Here's how the part is built. I have some questions about the finished solid (model axes, mm). A direction names the side the tool comes from. Round coordinates to 2 decimals unless told otherwise and drop trailing zeros. Order: outer loops, then holes, each group sorted by start corner. A loop starts at its lowest first (then second) coordinate and runs counter-clockwise, first axis right, second up. Notation, with made-up numbers: (71.25, 10.5) -> (125.25, 10.5) arc R36 ccw to (125.25, 48.5) -> close; hole circle Ø7 at (-1.75, 87). An arc over 180 degrees is marked (long way). One line per item, written item: value.
```python
from build123d import *

# Parameters (mm, degrees)
SKETCH_1_R          = 8
EXTRUDE_1_DEPTH     = 10
SKETCH_2_R          = 5
EXTRUDE_2_DEPTH     = 42
SKETCH_3_R          = 3.5
EXTRUDE_3_DEPTH     = 12
CUT_EXTRUDE_1_DEPTH = 10


with BuildPart() as part:
    # Эскиз1 → Бобышка-Вытянуть1 (new body)
    with BuildSketch(Plane(origin=(0, 0, 0), x_dir=(1, 0, 0), z_dir=(0, 1, 0))):
        Circle(SKETCH_1_R)
    extrude(amount=EXTRUDE_1_DEPTH)

    # Эскиз2 → Бобышка-Вытянуть2 (add)
    with BuildSketch(Plane(origin=(0, 10, 0), x_dir=(1, 0, 0), z_dir=(0, 1, 0))):
        Circle(SKETCH_2_R)
    extrude(amount=EXTRUDE_2_DEPTH)

    # Эскиз3 → Бобышка-Вытянуть3 (add)
    with BuildSketch(Plane(origin=(0, 52, 0), x_dir=(1, 0, 0), z_dir=(0, 1, 0))):
        Circle(SKETCH_3_R)
    extrude(amount=EXTRUDE_3_DEPTH)

    # Эскиз4 → Вырез-Вытянуть1 (cut)
    with BuildSketch(Plane(origin=(0, 0, 0), x_dir=(0, 0, -1), z_dir=(1, 0, 0))):
        with BuildLine():
            Line((-2, 42), (-2, 48))
            ThreePointArc((-2, 48), (0, 50), (2, 48))
            Line((2, 48), (2, 42))
            ThreePointArc((2, 42), (0, 40), (-2, 42))
        make_face()
    extrude(amount=-CUT_EXTRUDE_1_DEPTH, mode=Mode.SUBTRACT)


solid = part.part
```
Q1. I want a section at C-C on y = 7. Write out the boundary of the cut face in (x, z), then the cut area to 3 significant figures.
Answers:
outline: circle Ø16 at (0, 0)
area: 201 mm2
Q2. If we mould it in two halves opening along Z, with no side actions, what happens to faces 4 (the face through (0, 45, 0)), 5 (the face through (-2, 40, 0)), 6 (the face through (0, 64, 0)), 7 (the face through (4.77, 30.71, -1.5))? For each: pulls with the +Z half, pulls with the -Z half, needs draft (parallel to the pull), parting line crosses it, or undercut.
Answers:
face 4: undercut
face 5: undercut
face 6: needs draft
face 7: parting line crosses it
Q3. I need wall thicknesses on line 1 along Y through (x, z) = (-2.5, 3.5); line 2 along Y through (x, z) = (7.5, 0); line 3 along X through (y, z) = (7, -3.5). Which ranges of each line are inside material? Lowest first, please.
Answers:
line 1: 0 to 52
line 2: 0 to 10
line 3: -7.19 to 7.19
Q4. Which directions (+Z, -Z, +X, -X, +Y, -Y) give clear straight access to the entire face, cutting with the end or side of a thin tool? Please do faces 1 (the face through (-2, 45, -2)), 2 (the face through (0, 0, 0)), 3 (the face through (5.2, 10, -0.1)).
Answers:
face 1: -X
face 2: +Z, -Z, +X, -X, -Y
face 3: +Y
Q5. I want a section at D-D on z = 6. Write out the boundary of the cut face in (x, y), then the cut area to 3 significant figures.
Answers:
outline: (-5.29, 0) -> (5.29, 0) -> (5.29, 10) -> (-5.29, 10) -> close
area: 106 mm2
Q6. I want a section at B-B on x = -2.5. Write out the boundary of the cut face in (y, z).
Answers:
outline: (0, -7.6) -> (10, -7.6) -> (10, -4.33) -> (52, -4.33) -> (52, -2.45) -> (64, -2.45) -> (64, 2.45) -> (52, 2.45) -> (52, 4.33) -> (10, 4.33) -> (10, 7.6) -> (0, 7.6) -> close; hole (42, -2) -> (48, -2) arc R2 ccw to (48, 2) -> (42, 2) arc R2 ccw to start
Q7. I want a section at A-A on z = 0. Write out the boundary of the cut face in (x, y), then the cut area to 3 significant figures.
Answers:
outline: (-8, 0) -> (8, 0) -> (8, 10) -> (5, 10) -> (5, 52) -> (3.5, 52) -> (3.5, 64) -> (-3.5, 64) -> (-3.5, 52) -> (-5, 52) -> (-5, 50) -> (0, 50) -> (0, 40) -> (-5, 40) -> (-5, 10) -> (-8, 10) -> close
area: 614 mm2
Q8. For P1, Ø5, axis at x = -1.5, y = 44.5, coming from the -Z side; P2, Ø4.5, axis at y = 47, z = 0, coming from the -X side; P3, Ø8, axis at x = -5.5, y = 35.5, coming from the -Z side, each with a flat end and sliding along its axis, tell me the tip position at first contact or that it passes through.
Answers:
P1: z = -5
P2: x = -4.58
P3: z = -4.77
